Verification items for the finished model (mm, model axes). Face numbers are marked on the shaded views. A direction names the side the tool comes from. Coordinates: 2 decimals unless noted, no trailing zeros. Order: outer loops, then holes, each group sorted by start corner. A loop starts at its lowest first (then second) coordinate and runs counter-clockwise, first axis right, second up. Notation, with made-up numbers: (28.5, -7.5) -> (76.5, -7.5) arc R23 cw to (76.5, 17.5) -> close; hole circle Ø2 at (78.25, -10.75). An arc over 180 degrees is marked (long way). Write item = value, one per line. Start each with the question number.
1. Go/stop test with flat-tipped pins: P1, Ø10, axis at x = 62.6, y = -51.42, coming from the +Z side; P2, Ø1.5, axis at y = -30.5, z = 4.5, coming from the -X side; P3, Ø1.5, axis at y = -50, z = 1.5, coming from the +X side; P4, Ø1, axis at y = -36.5, z = 2.5, coming from the -X side. Record where each tip stops, or that it passes through.
2. Release check for a two-part mould opening along X. For the marked faces 1, 2 and 3 record: +X half, -X half, draft (parallel to the pull), parting line (faces both ways), or undercut.
3. Thickness scan on line 1 along Y through (x, z) = (39, 5.5); line 2 along Y through (x, z) = (40.5, 4); line 3 along X through (y, z) = (-35, 6). Record the ranges inside material, lowest first. Write a range as from..to.
4. Cross-section at B-B on x = 28. Record the cut outline in (y, z), plus the area to 3 significant figures.
5. Cross-section at A-A on y = -27. Record the cut outline in (x, z), plus the area to 3 significant figures.
6. Cross-section at C-C on z = 5. Give the number of separate pieces and of enclosed holes in the cut face, plus the area to 3 significant figures.
7. Cross-section at D-D on y = -11.5. Record the cut outline in (x, z).
8. Set-up check for the marked faces 4 and 5: record each of +Z, -Z, +X, -X, +Y, -Y from which the full face is reachable in a straight line by a thin tool's end or side.
from build123d import *

# Parameters (mm, degrees)
SKETCH1_R           = 4.7625
BOSS_EXTRUDE1_DEPTH = 6.35
BOSS_EXTRUDE2_START = -6.35
SKETCH2_R           = 4.7625
SKETCH2_R_2         = 3.175
BOSS_EXTRUDE2_DEPTH = 6.35
CUT_EXTRUDE1_DEPTH  = 6.35


with BuildPart() as part:
    # Sketch1 → Boss-Extrude1 (new body)
    with BuildSketch(Plane.XY):
        with BuildLine():
            Line((31.405613519, -6.275848049), (7.910613519, -46.970381773))
            ThreePointArc((7.910613519, -46.970381773), (7.910613519, -55.860381773), (15.609579358, -60.305381773))
            Line((15.609579358, -60.305381773), (62.599579358, -60.305381773))
            ThreePointArc((62.599579358, -60.305381773), (70.298545198, -55.860381773), (70.298545198, -46.970381773))
            Line((70.298545198, -46.970381773), (46.803545198, -6.275848049))
            ThreePointArc((46.803545198, -6.275848049), (39.104579358, -1.830848049), (31.405613519, -6.275848049))
        make_face()
        with Locations((39.073094298, -10.775381773)):
            Circle(SKETCH1_R, mode=Mode.SUBTRACT)
        with Locations((15.609579358, -51.415381773)):
            Circle(SKETCH1_R, mode=Mode.SUBTRACT)
        with Locations((62.599579358, -51.415381773)):
            Circle(SKETCH1_R, mode=Mode.SUBTRACT)
        with BuildLine():
            Line((36.904874833, -22.150848049), (24.408397461, -43.795381773))
            ThreePointArc((24.408397461, -43.795381773), (24.408397461, -46.335381773), (26.608101987, -47.605381773))
            Line((26.608101987, -47.605381773), (51.60105673, -47.605381773))
            ThreePointArc((51.60105673, -47.605381773), (53.800761256, -46.335381773), (53.800761256, -43.795381773))
            Line((53.800761256, -43.795381773), (41.304283884, -22.150848049))
            ThreePointArc((41.304283884, -22.150848049), (39.104579358, -20.880848049), (36.904874833, -22.150848049))
        make_face(mode=Mode.SUBTRACT)
    extrude(amount=BOSS_EXTRUDE1_DEPTH)

    # Sketch2 → Boss-Extrude2 (add)
    # profile 1 of 3: a face of its own
    with BuildSketch(Plane.XY.offset(6.35).offset(BOSS_EXTRUDE2_START)):
        with Locations((39.073094298, -10.775381773)):
            Circle(SKETCH2_R)
        with Locations((39.073094298, -10.775381773)):
            Circle(SKETCH2_R_2, mode=Mode.SUBTRACT)
    # profile 2 of 3: a face of its own
    with BuildSketch(Plane.XY.offset(6.35).offset(BOSS_EXTRUDE2_START)):
        with Locations((62.599579358, -51.415381773)):
            Circle(SKETCH2_R)
        with Locations((62.599579358, -51.415381773)):
            Circle(SKETCH2_R_2, mode=Mode.SUBTRACT)
    # profile 3 of 3: a face of its own
    with BuildSketch(Plane.XY.offset(6.35).offset(BOSS_EXTRUDE2_START)):
        with Locations((15.609579358, -51.415381773)):
            Circle(SKETCH2_R)
        with Locations((15.609579358, -51.415381773)):
            Circle(SKETCH2_R_2, mode=Mode.SUBTRACT)
    extrude(amount=BOSS_EXTRUDE2_DEPTH)

    # Sketch3 → Cut-Extrude1 (cut)
    with BuildSketch(Plane.XY.offset(6.35)):
        with BuildLine():
            Line((17.432559504, -40.002887539), (30.132559504, -18.005842283))
            ThreePointArc((30.132559504, -18.005842283), (32.301124833, -17.424776955), (32.882190161, -19.593342283))
            Line((32.882190161, -19.593342283), (20.182190161, -41.590387539))
            ThreePointArc((20.182190161, -41.590387539), (18.013624833, -42.171452868), (17.432559504, -40.002887539))
        make_face()
        with BuildLine():
            Line((48.048040695, -18.005842283), (60.748040695, -40.002887539))
            ThreePointArc((60.748040695, -40.002887539), (60.166975366, -42.171452868), (57.998410038, -41.590387539))
            Line((57.998410038, -41.590387539), (45.298410038, -19.593342283))
            ThreePointArc((45.298410038, -19.593342283), (45.879475366, -17.424776955), (48.048040695, -18.005842283))
        make_face()
        with BuildLine():
            Line((51.790300099, -55.518149371), (26.390300099, -55.518149371))
            ThreePointArc((26.390300099, -55.518149371), (24.802800099, -53.930649371), (26.390300099, -52.343149371))
            Line((26.390300099, -52.343149371), (51.790300099, -52.343149371))
            ThreePointArc((51.790300099, -52.343149371), (53.377800099, -53.930649371), (51.790300099, -55.518149371))
        make_face()
    extrude(amount=-CUT_EXTRUDE1_DEPTH, mode=Mode.SUBTRACT)


solid = part.part
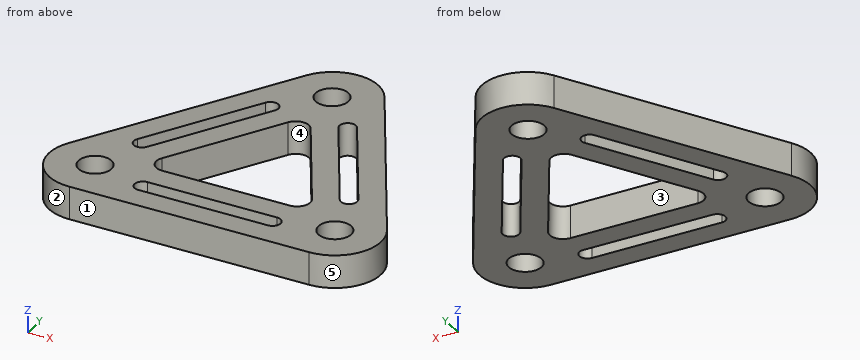
Worked out:
q1.P1 = 6.35
q1.P2 = 16.99
q1.P3 = 71.46
q1.P4 = 13.67
q2.face_1 = draft
q2.face_2 = -X half
q2.face_3 = undercut
q3.line_1 = -60.31..-55.52, -52.34..-47.61, -20.88..-13.95, -7.6..-1.83
q3.line_2 = -60.31..-55.52, -52.34..-47.61, -21.3..-13.61, -7.94..-1.94
q3.line_3 = 14.82..20.32, 23.99..29.49, 48.72..54.19, 57.86..63.39
q4.outline = (-60.31, 0) -> (-55.52, 0) -> (-55.52, 6.35) -> (-60.31, 6.35) -> close; (-52.34, 0) -> (-47.61, 0) -> (-47.61, 6.35) -> (-52.34, 6.35) -> close; (-37.57, 0) -> (-28.05, 0) -> (-28.05, 6.35) -> (-37.57, 6.35) -> close; (-21.7, 0) -> (-12.17, 0) -> (-12.17, 6.35) -> (-21.7, 6.35) -> close
q4.area = 181 mm²
q5.outline = (19.44, 0) -> (24.94, 0) -> (24.94, 6.35) -> (19.44, 6.35) -> close; (28.61, 0) -> (34.11, 0) -> (34.11, 6.35) -> (28.61, 6.35) -> close; (44.1, 0) -> (49.57, 0) -> (49.57, 6.35) -> (44.1, 6.35) -> close; (53.24, 0) -> (58.77, 0) -> (58.77, 6.35) -> (53.24, 6.35) -> close
q5.area = 140 mm²
q6.separate_pieces = 1
q6.enclosed_holes = 7
q6.area = 1,620 mm²
q7.outline = (28.39, 0) -> (35.98, 0) -> (35.98, 6.35) -> (28.39, 6.35) -> close; (42.16, 0) -> (49.82, 0) -> (49.82, 6.35) -> (42.16, 6.35) -> close
q8.face_4 = +Z, -Z
q8.face_5 = +Z, -Z, +X
